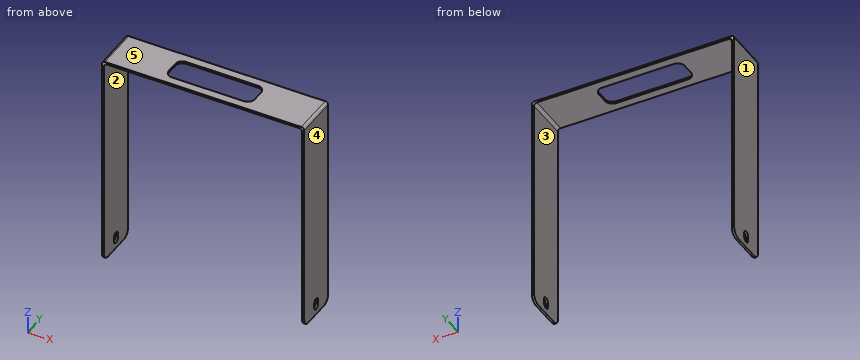
from build123d import *

# Parameters (mm, degrees)
F0_W     = 141
F0_H     = 30
F0_W_2   = 60
F0_H_2   = 18
F1_DEPTH = 1.5
F2_W     = 1.5
F2_H     = 30
F3_DEPTH = 150
F4_R     = 5
F7_DEPTH = 200
F8_R     = 2


# Not quite as in the source:
# - two fillets or chamfers of one size are made in one step


with BuildPart() as f1:
    # F0 (on Top) → F1 (new body)
    with BuildSketch(Plane.XY):
        Rectangle(F0_W, F0_H)
        Rectangle(F0_W_2, F0_H_2, mode=Mode.SUBTRACT)
    extrude(amount=F1_DEPTH)

    # F2 (on face) → F3 (join)
    with BuildSketch(Plane(origin=(0, 0, 0), x_dir=(1, 0, 0), z_dir=(0, 0, -1))):
        with Locations((-69.75, 0)):
            Rectangle(F2_W, F2_H)
        with Locations((69.75, 0)):
            Rectangle(F2_W, F2_H)
    extrude(amount=F3_DEPTH)

    # F4
    f4_edges = [f1.edges().sort_by_distance(p)[0] for p in [
        (30, 9, 0.75),
        (30, -9, 0.75),
        (-30, -9, 0.75),
        (-30, 9, 0.75),
        (-69.75, 15, -150),
        (69.75, 15, -150),
        (69.75, -15, -150),
        (-69.75, -15, -150),
    ]]
    fillet(f4_edges, radius=F4_R)

    # F6 (on face) → F7 (cut)
    with BuildSketch(Plane(origin=(-70.5, 0, 0), x_dir=(0, -1, 0), z_dir=(-1, 0, 0))):
        with BuildLine():
            Line((-2.5, -140.5), (-2.5, -143.5))
            ThreePointArc((-2.5, -143.5), (-1.767766953, -145.267766953), (0, -146))
            ThreePointArc((0, -146), (1.767766953, -145.267766953), (2.5, -143.5))
            Line((2.5, -143.5), (2.5, -140.5))
            ThreePointArc((2.5, -140.5), (1.767766953, -138.732233047), (0, -138))
            ThreePointArc((0, -138), (-1.767766953, -138.732233047), (-2.5, -140.5))
        make_face()
    extrude(amount=-F7_DEPTH, mode=Mode.SUBTRACT)

    # F8
    f8_edges = [f1.edges().sort_by_distance(p)[0] for p in [
        (70.5, 0, 1.5),
        (-70.5, 0, 1.5),
        (-69, 0, 0),
        (69, 0, 0),
    ]]
    fillet(f8_edges, radius=F8_R)


solid = f1.part
Can you work these out from the model? Positions are in its coordinate system, mm. Face numbers are marked on the shaded views. A direction names the side the tool comes from. Coordinates: 2 decimals unless noted, no trailing zeros. Order: outer loops, then holes, each group sorted by start corner. A loop starts at its lowest first (then second) coordinate and runs counter-clockwise, first axis right, second up. Notation, with made-up numbers: (28.25, 59.5) - (37.25, 59.5) arc R7 cw to (37.25, 67.5) - close; hole circle Ø6 at (-30, 40.25). An arc over 180 degrees is marked (long way). Answer as a JSON object with one key per item and string values. Group by question number.
Q1. Imagine slicing it at D-D (x = -42.5). Please give me the cut outline in (y, z).
Q2. Imagine slicing it at B-B (z = -113.5). Please give me the cut outline in (x, y).
Q3. Imagine slicing it at A-A (x = -13.5). Please give me the cut outline in (y, z).
Q4. Imagine slicing it at C-C (y = 6). Please give me the cut outline in (x, z).
Q5. We'd pull the mould along X, two halves only. Please class the marked faces 3, 4 and 5: +X half, -X half, draft (parallel to the pull), parting line (faces both ways), or undercut.
Q6. On a 3-axis mill with a long thin cutter (end or side, diameter ignored), from which of +Z, -Z, +X, -X, +Y, -Y can I reach the whole of each face in a straight line? I mean the marked faces 1 and 2. Say none if no direction works.
Q7. Will these pins go through, and if not, where does the flat tip stop? P1, Ø0.8, axis at y = -0.5, z = 1, coming from the +X side; P2, Ø5, axis at x = -48, y = 0.5, coming from the -Z side; P3, Ø1.2, axis at y = -1.5, z = 0.5, coming from the -X side.
Q8. I need wall thicknesses on line 1 (X direction, y = -2.75, z = -88.5); line 2 (Z direction, x = 36.5, y = -7.5). Which ranges of each line are inside material? Lowest first, please. Write a range as from..to.
Determined:
{
 "1": {"outline": "(-15, 0) - (15, 0) - (15, 1.5) - (-15, 1.5) - close"},
 "2": {"outline": "(-70.5, -15) - (-69, -15) - (-69, 15) - (-70.5, 15) - close; (69, -15) - (70.5, -15) - (70.5, 15) - (69, 15) - close"},
 "3": {"outline": "(-15, 0) - (-9, 0) - (-9, 1.5) - (-15, 1.5) - close; (9, 0) - (15, 0) - (15, 1.5) - (9, 1.5) - close"},
 "4": {"outline": "(-70.5, -150) - (-69, -150) - (-69, -2) arc R2 cw to (-67, 0) - (-29.58, 0) - (-29.58, 1.5) - (-68.5, 1.5) arc R2 ccw to (-70.5, -0.5) - close; (29.58, 0) - (67, 0) arc R2 cw to (69, -2) - (69, -150) - (70.5, -150) - (70.5, -0.5) arc R2 ccw to (68.5, 1.5) - (29.58, 1.5) - close"},
 "5": {"face 3": "undercut", "face 4": "+X half", "face 5": "draft"},
 "6": {"face 1": "+Z, -Z, -X, +Y, -Y", "face 2": "-Z, +Y, -Y"},
 "7": {"P1": "stops at x = 70.17", "P2": "stops at z = 0", "P3": "stops at x = -70.46"},
 "8": {"line 1": "x = -70.5..-69, 69..70.5", "line 2": "z = 0..1.5"}
}
